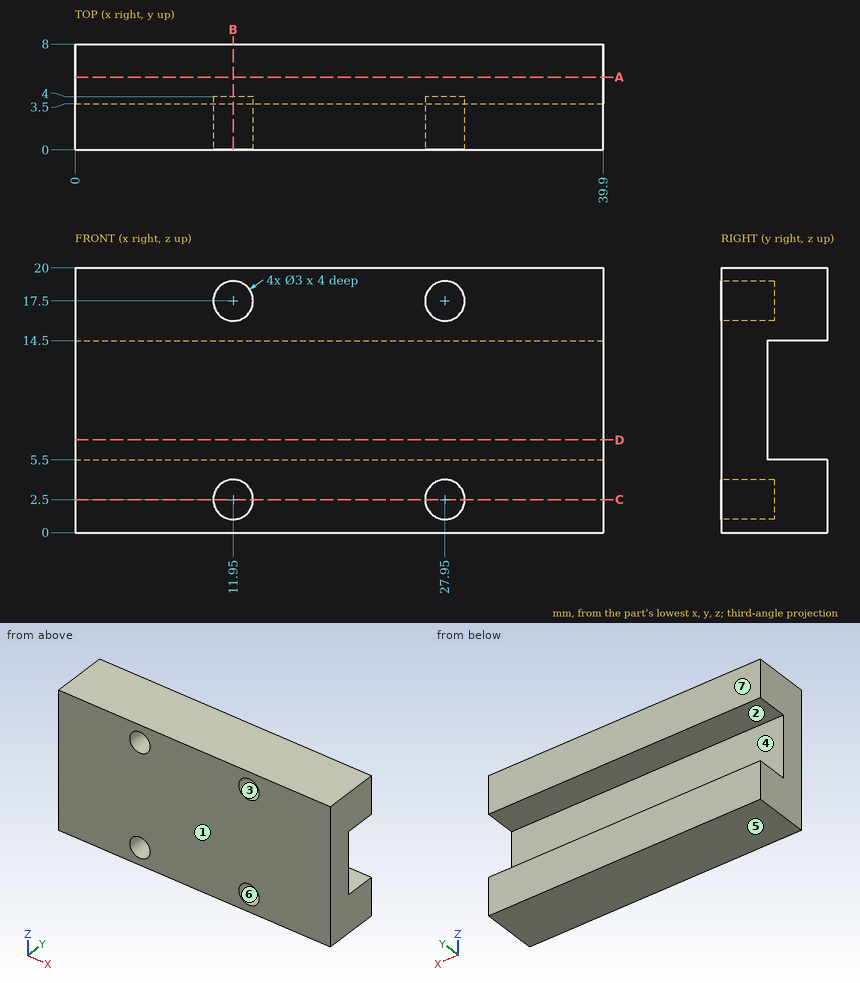
Drawing for the job (mm, zero at the part's lowest x, y, z). A direction names the side the tool comes from. Round coordinates to 2 decimals unless told otherwise and drop trailing zeros. Loops run counter-clockwise (first coordinate to the right, second up) from the corner with the lowest first, then second, coordinate; pieces in that order, holes last.
1. Band-saw the part on D-D, the plane z = 7. List the corners of the cut face in (x, y).
Check values:
outline: (0, 0) - (39.9, 0) - (39.9, 3.5) - (0, 3.5) - close
2. Mould opens along Z. For the marked faces 4, 5, 6 and 7 say: +Z half, -Z half, draft (parallel to the pull), parting line (faces both ways), or undercut.
Check values:
face 4: undercut
face 5: -Z half
face 6: undercut
face 7: draft
3. Tool access for the marked faces 1, 2 and 3: list every direction of +Z, -Z, +X, -X, +Y, -Y with a clear straight run to the whole face (end or side of a thin tool).
Check values:
face 1: +Z, -Z, +X, -X, -Y
face 2: +X, -X, +Y
face 3: -Y
4. Band-saw the part on B-B, the plane x = 11.95. List the corners of the cut face in (y, z), and give its area (3 significant figures).
Check values:
outline: (0, 0) - (8, 0) - (8, 5.5) - (3.5, 5.5) - (3.5, 14.5) - (8, 14.5) - (8, 20) - (0, 20) - (0, 19) - (4, 19) - (4, 16) - (0, 16) - (0, 4) - (4, 4) - (4, 1) - (0, 1) - close
area: 95.5 mm2
5. Drop flat-ended pins along their axis: P1, Ø0.9, axis at x = 27.5, z = 18, coming from the -Y side; P2, Ø2, axis at x = 24, z = 7, coming from the +Y side. Give the stop position or say it passes through.
Check values:
P1: stops at y = 4
P2: stops at y = 3.5
6. Wall check: probe 1 along Z at (x, y) = (11.95, 1.3); probe 2 along Z at (x, y) = (6, 7.75); probe 3 along Y at (x, z) = (21, 11). Give the ranges that are in metal, low to high.
Check values:
probe 1: z = 0 to 1, 4 to 16, 19 to 20
probe 2: z = 0 to 5.5, 14.5 to 20
probe 3: y = 0 to 3.5
7. Band-saw the part on A-A, the plane y = 5.5. List the corners of the cut face in (x, z).
Check values:
outline: (0, 0) - (39.9, 0) - (39.9, 5.5) - (0, 5.5) - close; (0, 14.5) - (39.9, 14.5) - (39.9, 20) - (0, 20) - close
8. Band-saw the part on C-C, the plane z = 2.5. List the corners of the cut face in (x, y).
Check values:
outline: (0, 0) - (10.45, 0) - (10.45, 4) - (13.45, 4) - (13.45, 0) - (26.45, 0) - (26.45, 4) - (29.45, 4) - (29.45, 0) - (39.9, 0) - (39.9, 8) - (0, 8) - close
